Here's how the part is built. I have some questions about the finished solid (model axes, mm). A direction names the side the tool comes from. Round coordinates to 2 decimals unless told otherwise and drop trailing zeros. Loops run counter-clockwise (first coordinate to the right, second up) from the corner with the lowest first, then second, coordinate; pieces in that order, holes last. Notation, with made-up numbers: (2, -10.75) - (35, -10.75) arc R18 cw to (35, 5.25) - close; hole circle Ø8 at (-25, 38.25). An arc over 180 degrees is marked (long way). Answer as a JSON object with one key per item and string values. Group by question number.
1) Which directions (+Z, -Z, +X, -X, +Y, -Y) give clear straight access to the entire face, cutting with the end or side of a thin tool? Please do faces 1 (the face through (-27.5, -1, 10)), 2 (the face through (-9, -9, 31)), 3 (the face through (-15, 16, 43)), 4 (the face through (-8.4, -4, 21.8)), 5 (the face through (-9, 41, 31)).
2) Will these pins go through, and if not, where does the flat tip stop? P1, Ø12, axis at x = 15.5, y = -38, coming from the -Z side; P2, Ø2, axis at x = -12, z = 33, coming from the -Y side; P3, Ø12, axis at x = 20.5, y = 36, coming from the +Z side; P4, Ø10, axis at x = -8, z = 26.5, coming from the +Y side.
3) I want a section at B-B, the plane y = -38. Please give me the cut outline in (x, z), then the cut area to 3 significant figures.
4) I want a section at A-A, the plane x = -8.5. Please give me the cut outline in (y, z).
5) I want a section at C-C, the plane z = 13. Please give me the cut outline in (x, y).
6) If we mould it in two halves opening along X, with no side actions, what happens to faces 6 (the face through (-18.5, 16, 31)), 7 (the face through (1.5, 16, 31)), 8 (the face through (-8.6, 36, 21.8))? For each: pulls with the +X half, pulls with the -X half, needs draft (parallel to the pull), parting line crosses it, or undercut.
7) If I drill on line 1 along Y through (x, z) = (15.5, 15.75); line 2 along X through (y, z) = (10, 19); line 3 along X through (y, z) = (39, 40.5), over which ranges is the centre line in solid material (lowest first)? Write a range as [from, to].
8) I want a section at D-D, the plane z = 39.5. Please give me the cut outline in (x, y).
from build123d import *

# Parameters (mm, degrees)
SKETCH_1_W          = 55
SKETCH_1_H          = 100
EXTRUDE_1_DEPTH     = 20
SKETCH_2_R          = 7.5
CUT_EXTRUDE_1_DEPTH = 61.466933112
SKETCH_3_W          = 20
SKETCH_3_H          = 50
EXTRUDE_2_DEPTH     = 23
CUT_EXTRUDE_2_DEPTH = 72.451032183


with BuildPart() as part:
    # Эскиз1 → Бобышка-Вытянуть1 (new body)
    with BuildSketch(Plane.XY):
        Rectangle(SKETCH_1_W, SKETCH_1_H)
    extrude(amount=EXTRUDE_1_DEPTH)

    # Эскиз2 → Вырез-Вытянуть1 (cut, through all)
    with BuildSketch(Plane.XY.offset(20)):
        with Locations((15.5, -38)):
            Circle(SKETCH_2_R)
    extrude(amount=-CUT_EXTRUDE_1_DEPTH, mode=Mode.SUBTRACT)

    # Эскиз3 → Бобышка-Вытянуть2 (add)
    with BuildSketch(Plane.XY.offset(20)):
        with Locations((-8.5, 16)):
            Rectangle(SKETCH_3_W, SKETCH_3_H)
    extrude(amount=EXTRUDE_2_DEPTH)

    # Эскиз4 → Вырез-Вытянуть2 (cut, through all)
    with BuildSketch(Plane.XY.offset(43)):
        with BuildLine():
            Line((-14.5, 2), (-14.5, 30))
            ThreePointArc((-14.5, 30), (-8.5, 36), (-2.5, 30))
            Line((-2.5, 30), (-2.5, 2))
            ThreePointArc((-2.5, 2), (-8.5, -4), (-14.5, 2))
        make_face()
    extrude(amount=-CUT_EXTRUDE_2_DEPTH, mode=Mode.SUBTRACT)


solid = part.part
Outcome:
{
 "1": {"face 1": "+Z, -Z, -X, +Y, -Y", "face 2": "+Z, +X, -X, -Y", "face 3": "+Z, +X, -X, +Y, -Y", "face 4": "+Z, -Z", "face 5": "+Z, +X, -X, +Y"},
 "2": {"P1": "through", "P2": "y = -9", "P3": "z = 20", "P4": "y = 41"},
 "3": {"outline": "(-27.5, 0) - (8, 0) - (8, 20) - (-27.5, 20) - close; (23, 0) - (27.5, 0) - (27.5, 20) - (23, 20) - close", "area": "800 mm^2"},
 "4": {"outline": "(-50, 0) - (-4, 0) - (-4, 43) - (-9, 43) - (-9, 20) - (-50, 20) - close; (36, 0) - (50, 0) - (50, 20) - (41, 20) - (41, 43) - (36, 43) - close"},
 "5": {"outline": "(-27.5, -50) - (27.5, -50) - (27.5, 50) - (-27.5, 50) - close; hole (-14.5, 2) arc R6 ccw to (-2.5, 2) - (-2.5, 30) arc R6 ccw to (-14.5, 30) - close; hole circle Ø15 at (15.5, -38)"},
 "6": {"face 6": "pulls with the -X half", "face 7": "pulls with the +X half", "face 8": "undercut"},
 "7": {"line 1": "[-50, -45.5], [-30.5, 50]", "line 2": "[-27.5, -14.5], [-2.5, 27.5]", "line 3": "[-18.5, 1.5]"},
 "8": {"outline": "(-18.5, -9) - (1.5, -9) - (1.5, 41) - (-18.5, 41) - close; hole (-14.5, 2) arc R6 ccw to (-2.5, 2) - (-2.5, 30) arc R6 ccw to (-14.5, 30) - close"}
}
